```python
from build123d import *

# Parameters (mm, degrees)
EXTRUDE_BASE_DEPTH              = 30
SKETCH2_R                       = 2.2
CUT_BOLT_HOLES_DEPTH            = 10
CUT_BOLT_HEAD_INSETS_DEPTH      = 40
CUT_BOLT_HEAD_INSETS_DEPTH_BACK = 4.2
SKETCH3_R                       = 4.215
SKETCH4_W                       = 40
SKETCH4_H                       = 3
CUT_TOP_CLEARANCE_SLOT_DEPTH    = 45
FILLET_CLEARANCE_SLOT_PT_1_R    = 3
FILLET_CLEARANCE_SLOT_PT_2_R    = 3


# Some blends are built 0.0001 mm under size
with BuildPart() as part:
    # Sketch1 → Extrude-Base (new, symmetric)
    with BuildSketch(Plane.XY):
        Polygon((-14, 0), (0, 0), (0, -35), (-98, -35), (-98, -29), (-83, -29), (-83, -13), (-90, -13), (-90, -9), (-79, -9), (-79, -29), (-4, -29), (-4, -4), (-14, -4), align=None)
    extrude(amount=EXTRUDE_BASE_DEPTH, both=True)

    # Sketch2 → Cut-Bolt Holes (cut)
    with BuildSketch(Plane(origin=(0, -29, 0), x_dir=(1, 0, 0), z_dir=(0, 1, 0))):
        with Locations(Location((-15, -10, 0), (0, 0, 270))):
            Circle(SKETCH2_R)
        with Locations(Location((-15, 10, 0), (0, 0, 270))):
            Circle(SKETCH2_R)
        with Locations(Location((-35, 10, 0), (0, 0, 270))):
            Circle(SKETCH2_R)
        with Locations(Location((-35, -10, 0), (0, 0, 270))):
            Circle(SKETCH2_R)
    extrude(amount=-CUT_BOLT_HOLES_DEPTH, mode=Mode.SUBTRACT)

    # Sketch3 → Cut-Bolt Head Insets (cut, two sides: drawn at the far end of the back side and taken through both)
    with BuildSketch(Plane(origin=(0, -29, 0), x_dir=(1, 0, 0), z_dir=(0, 1, 0)).offset(-CUT_BOLT_HEAD_INSETS_DEPTH_BACK)):
        with Locations((-35, 10)):
            Circle(SKETCH3_R)
        with Locations((-15, 10)):
            Circle(SKETCH3_R)
        with Locations((-15, -10)):
            Circle(SKETCH3_R)
        with Locations((-35, -10)):
            Circle(SKETCH3_R)
    extrude(amount=CUT_BOLT_HEAD_INSETS_DEPTH + CUT_BOLT_HEAD_INSETS_DEPTH_BACK, mode=Mode.SUBTRACT)

    # Sketch4 → Cut-Top Clearance Slot (cut)
    with BuildSketch(Plane.ZY.offset(98)):
        with Locations((0, -33.5)):
            Rectangle(SKETCH4_W, SKETCH4_H)
    extrude(amount=-CUT_TOP_CLEARANCE_SLOT_DEPTH, mode=Mode.SUBTRACT)

    # Fillet-Clearance Slot Pt 1
    fillet_clearance_slot_pt_1_edges = [part.edges().sort_by_distance(p)[0] for p in [
        (-75.5, -32, 20),
        (-75.5, -32, -20),
    ]]
    fillet(fillet_clearance_slot_pt_1_edges, radius=FILLET_CLEARANCE_SLOT_PT_1_R - 0.0001)  # a hair under: the kernel refuses the full size

    # Fillet-Clearance Slot Pt 2
    # the kernel refuses this fillet: 3 mm, written as the material it takes off along each edge
    with BuildSketch(Plane(origin=(-103.490486718, -35, 20), x_dir=(0, 0, 1), z_dir=(1, 0, 0))) as fillet_clearance_slot_pt_2_piece_1:
        with BuildLine():
            CenterArc((2.196194687, -3), FILLET_CLEARANCE_SLOT_PT_2_R, 90, 60.000551337)
            Line((-0.401895958, -1.500025), (-0.661705022, -1.3500275))
            ThreePointArc((-0.661705022, -1.3500275), (-0.3, -0.0001), (-0.3, 0))
            Line((-0.3, 0), (0, 0.3))
            Line((0, 0.3), (2.196194687, 0.3))
            Line((2.196194687, 0.3), (2.196194687, 0))
        make_face()
    extrude(amount=50.490486718, mode=Mode.SUBTRACT)
    with BuildSketch(Plane(origin=(-103.490486718, -35, -20), x_dir=(0, 0.9659313848535176, 0.25879829936644777), z_dir=(1, 0, 0))) as fillet_clearance_slot_pt_2_piece_2:
        with BuildLine():
            CenterArc((2.329422704, -2.897768274), FILLET_CLEARANCE_SLOT_PT_2_R, 105.000679234, 60.000551337)
            Line((-0.56837145, -2.121373376), (-0.858150866, -2.043733886))
            Line((-0.858150866, -2.043733886), (-0.289779415, 0.07763949))
            Line((-0.289779415, 0.07763949), (0.07763949, 0.289779415))
            ThreePointArc((0.07763949, 0.289779415), (0.077736083, 0.289753536), (1.475282068, 0.289776827))
            Line((1.475282068, 0.289776827), (1.552931216, 0))
        make_face()
    extrude(amount=50.490486718, mode=Mode.SUBTRACT)


solid = part.part
```
Model file for the job. Use its own axes, mm. A direction names the side the tool comes from. Give positions to 0.01 mm unless a question says otherwise; leave off trailing zeros. Write each loop counter-clockwise with the first axis right and the second up, starting at its lowest first coordinate (ties: lowest second). Pieces come first, ordered by that corner, then holes. Notation, with made-up numbers: M -36,62 L 11,62 A16 cw 11,90 Z; hole C -38.75,-2 d5. An arc over 180 degrees is marked long. Use a Markdown table: item, result.
1) Pin check, flat tips, straight feed: pin 1 (5 mm diameter, centred on y = -15, z = -2, fed in from -X); pin 2 (1.5 mm diameter, centred on y = -8, z = -10, fed in from -X); pin 3 (17 mm diameter, centred on x = -80, z = -5.5, fed in from -Y); pin 4 (2.5 mm diameter, centred on x = -15, z = -10, fed in from +Y). Stop position of each tip, or through.
Responses:
| item | result |
|---|---|
| pin 1 | stops at x = -90 |
| pin 2 | stops at x = -4 |
| pin 3 | stops at y = -32 |
| pin 4 | passes through |
2) Pull direction Z, two halves, no side cores. Call faces 5 (the flat face through (-42, -29, 0)), 6 (the cylindrical face through (-75.8, -34.6, 20.7)), 7 (the flat face through (-45, -30, -30)): +Z half, -Z half, draft (parallel to the pull), parting line (faces both ways), or undercut.
Responses:
| item | result |
|---|---|
| face 5 | draft |
| face 6 | undercut |
| face 7 | -Z half |
3) Drill centre lines: line 1 (X direction, y = -34.3, z = 10); line 2 (Z direction, x = -15, y = -31.35) (3 decimals); line 3 (X direction, y = -29.9, z = 10) (3 decimals). Where is each one in solid material? Low to high. Write a range as from..to.
Responses:
| item | result |
|---|---|
| line 1 | x = -53..-37.2, -32.8..-17.2, -12.8..0 |
| line 2 | z = -30..-14.215, -5.785..5.785, 14.215..30 |
| line 3 | x = -98..-39.215, -30.785..-19.215, -10.785..0 |
4) Cut at B-B (z = -10). Give the number of separate pieces and of enclosed holes in the cut face, and give its area (3 significant figures).
Responses:
| item | result |
|---|---|
| separate pieces | 3 |
| enclosed holes | 0 |
| area | 617 mm2 |
5) Tool access for faces 1 (the flat face through (-14, -2, -22)), 2 (the cylindrical face through (-10.786, -2.028, 10.079)), 3 (the flat face through (-13, -33.2, 12)), 4 (the flat face through (-9, -4, 0)): list every direction of +Z, -Z, +X, -X, +Y, -Y with a clear straight run to the whole face (end or side of a thin tool).
Responses:
| item | result |
|---|---|
| face 1 | +Z, -Z, -X, +Y |
| face 2 | -X, +Y |
| face 3 | +Y |
| face 4 | +Z, -Z, -X |
6) Cut at A-A (y = -14). List the corners of the cut face in (x, z), and give its area (3 significant figures).
Responses:
| item | result |
|---|---|
| outline | M -83,-30 L -79,-30 L -79,30 L -83,30 Z; M -4,-30 L 0,-30 L 0,30 L -4,30 Z |
| area | 480 mm2 |
7) Cut at D-D (y = -1.5). List the corners of the cut face in (x, z) (3 decimals).
Responses:
| item | result |
|---|---|
| outline | M -14,-30 L 0,-30 L 0,30 L -14,30 L -14,14.095 A4.215 cw -14,5.905 L -14,-5.905 A4.215 cw -14,-14.095 Z |
8) Cut at C-C (x = -15). List the corners of the cut face in (y, z) (3 decimals).
Responses:
| item | result |
|---|---|
| outline | M -35,-30 L -29,-30 L -29,-14.215 L -33.2,-14.215 L -33.2,-12.2 L -35,-12.2 Z; M -35,-7.8 L -33.2,-7.8 L -33.2,-5.785 L -29,-5.785 L -29,5.785 L -33.2,5.785 L -33.2,7.8 L -35,7.8 Z; M -35,12.2 L -33.2,12.2 L -33.2,14.215 L -29,14.215 L -29,30 L -35,30 Z |
